Could you check a few things on this model? Use its own coordinates, in mm. A direction names the side the tool comes from. Give positions to 0.01 mm unless a question says otherwise; leave off trailing zeros. Write each loop counter-clockwise with the first axis right and the second up, starting at its lowest first coordinate (ties: lowest second). Pieces come first, ordered by that corner, then holes. Notation, with made-up numbers: M -14,26.5 L -4,26.5 A33 cw -4,64.5 Z; hole C 29.25,51.25 d5. An arc over 180 degrees is marked long. Answer as a JSON object with one key per item and string values. Group by question number.
```python
from build123d import *

# Parameters (mm, degrees)
F1_DEPTH = 63.5
F0_W     = 25.4
F0_H     = 19.05
F2_DEPTH = 25.4
F3_DEPTH = 7.9375


with BuildPart() as f1:
    # F0 (on Front) → F1 (new body, symmetric)
    with BuildSketch(Plane.XZ):
        Polygon((-90.502063, -9.525), (-7.952063, -9.525), (-7.952063, 9.525), (-27.002063, 9.525), (-90.502063, 9.525), align=None)
    extrude(amount=F1_DEPTH, both=True)

    # F0 (on Front) → F2 (join, symmetric)
    with BuildSketch(Plane.XZ):
        with BuildLine():
            Line((-27.002063, 9.525), (-7.952063, 9.525))
            Line((-7.952063, 9.525), (-7.952063, 27.0002))
            ThreePointArc((-7.952063, 27.0002), (-3.302383, 38.22552), (7.922937, 42.8752))
            Line((7.922937, 42.8752), (11.097937, 42.8752))
            Line((11.097937, 42.8752), (11.097937, 61.9252))
            Line((11.097937, 61.9252), (7.922937, 61.9252))
            add(Edge.make_bspline(
                [(1.660156, 61.359088), (3.749781, 61.58542), (5.838833, 61.774647), (7.922937, 61.9252)],
                knots=[106.639459, 106.639459, 106.639459, 106.639459, 111.504536, 111.504536, 111.504536, 111.504536], degree=3))
            ThreePointArc((1.660156, 61.359088), (-18.895743, 49.37237), (-27.002063, 27.0002))
            Line((-27.002063, 27.0002), (-27.002063, 9.525))
        make_face()
        with Locations((23.797937, 52.4002)):
            Rectangle(F0_W, F0_H)
    extrude(amount=F2_DEPTH, both=True)

    # F0 (on Front) → F3 (join, symmetric)
    with BuildSketch(Plane.XZ):
        with BuildLine():
            add(Edge.make_bspline(
                [(-90.502063, 9.525), (-90.221715, 33.60987), (-44.143125, 56.398042), (1.660156, 61.359088)],
                knots=[0, 0, 0, 0, 106.639459, 106.639459, 106.639459, 106.639459], degree=3))
            Line((-90.502063, 9.525), (-27.002063, 9.525))
            Line((-27.002063, 9.525), (-27.002063, 27.0002))
            ThreePointArc((-27.002063, 27.0002), (-18.895743, 49.37237), (1.660156, 61.359088))
        make_face()
    extrude(amount=F3_DEPTH, both=True)

    # F0 (on Front) → F4 (revolve)
    with BuildSketch(Plane.XZ):
        Polygon((36.497937, 61.9252), (36.497937, 42.8752), (36.497937, 38.1), (61.897937, 38.1), (61.897937, 66.675), (36.497937, 66.675), align=None)
    revolve(axis=Axis((36.497937, 0, 52.3875), (0, 0, -1)))


solid = f1.part
```
1) If we section it at A-A, the plane z = 7: List the corners of the cut face in (x, y) for me, plus the area to 3 significant figures.
2) I'm going to push flat-ended pins straight in: pin 1 (8.5 mm diameter, centred on y = -13.5, z = 21, fed in from -X); pin 2 (1 mm diameter, centred on x = -44, z = 28.5, fed in from +Y); pin 3 (12 mm diameter, centred on x = 43, y = -30.5, fed in from -Z). Where does each tip first touch, or does it pass through?
3) Please list where these lines run through material, in increasing order: line 1 along Z through (x, y) = (-18.5, 43) (3 decimals); line 2 along X through (y, z) = (35.5, -6); line 3 along Y through (x, z) = (-7.5, 51). Write a range as from..to.
4) If we section it at B-B, the plane y = 27.5: List the corners of the cut face in (x, z) for me (3 decimals), plus the area to 3 significant figures.
5) For faces 1 (the flat face through (-27.002, -17, 18)), 2 (the flat face through (-3, -25.4, 42)), 3 (the flat face through (37, 0, 38.1)), which set-ups out of +Z, -Z, +X, -X, +Y, -Y let a thin tool reach every point of the face, with its end or its side?
Taken from the geometry:
{
 "1": {"outline": "M -90.5,-63.5 L -7.95,-63.5 L -7.95,63.5 L -90.5,63.5 Z", "area": "10,500 mm²"},
 "2": {"pin 1": "x = -27", "pin 2": "y = 7.94", "pin 3": "z = 38.1"},
 "3": {"line 1": "-9.525..9.525", "line 2": "-90.5..-7.95", "line 3": "-25.4..25.4"},
 "4": {"outline": "M -90.502,-9.525 L -7.952,-9.525 L -7.952,9.525 L -90.502,9.525 Z", "area": "1,570 mm²"},
 "5": {"face 1": "+Z, -X, -Y", "face 2": "+Z, +X, -X, -Y", "face 3": "-Z, +X, +Y, -Y"}
}
